Work out the finished part from the listing and answer in its coordinate system (mm). A direction names the side the tool comes from. Coordinates: 2 decimals unless noted, no trailing zeros. Write each loop counter-clockwise with the first axis right and the second up, starting at its lowest first coordinate (ties: lowest second). Pieces come first, ordered by that corner, then holes. Notation, with made-up numbers: (16, 66) - (57, 66) arc R10 ccw to (57, 75) - close; hole circle Ø5 at (62, 3). An arc over 180 degrees is marked (long way). One line per item, written item: value.
Autodesk Inventor part; units mm, degrees
ref_plane "YZ Plane" through (0, 0, 0) normal (1, 0, 0) x (0, 1, 0)
ref_plane "XZ Plane" through (0, 0, 0) normal (0, 1, 0) x (-1, 0, 0)
ref_plane "XY Plane" through (0, 0, 0) normal (0, 0, 1) x (1, 0, 0)
sketch "Sketch1" plane through (0, 0, 0) normal (1, 0, 0) x (0, 1, 0)
  line L0 (22.5733, 37.2966) -> (14.6231, 37.2966)
  line L1 (14.6231, 37.2966) -> (14.6231, 5.5466)
  line L2 (14.6231, 5.5466) -> (22.5733, 5.5466)
  line L3 (22.5733, 5.5466) -> (22.5733, 37.2966)
  point P0 (0, 0)
  dimension "d0" = 7.9502
  dimension "d1" = 31.75
extrude "Extrusion1" add sketch "Sketch1" along normal blind 25.4
sketch "Sketch2" plane through (0, 14.6231, 37.2966) normal (0, 0, 1) x (1, 0, 0)
  line L0 (0, 7.9502) -> (25.4, 7.9502)
  line L1 (25.4, 0) -> (15.24, 0)
  line L2 (15.24, 0) -> (15.24, 7.9502)
  line L3 (15.24, 7.9502) -> (25.4, 7.9502)
  line L4 (25.4, 7.9502) -> (25.4, 0)
  point P0 (0, -14.6231)
  dimension "d4" = 10.16
extrude "Extrusion2" cut sketch "Sketch2" against normal blind 7.62
sketch "Sketch3" plane through (0, 14.6231, 29.6766) normal (0, 0, 1) x (1, 0, 0)
  line L0 (25.4, 7.9502) -> (25.4, 0)
  line L1 (15.24, 7.9502) -> (25.4, 7.9502)
  line L2 (15.24, 0) -> (15.24, 7.9502)
  line L3 (25.4, 0) -> (15.24, 0)
  circle A0 centre (20.32, 3.9502) radius 2
  point P0 (0, -14.6231)
  dimension "d7" = 4
  dimension "d10" = 4
extrude "Extrusion3" cut sketch "Sketch3" against normal blind 2.54 contours A0
sketch "Sketch4" plane through (0, 22.5733, 37.2966) normal (0, 1, 0) x (1, 0, 0)
  circle A0 centre (10.16, 6.0198) radius 2
  line L0 (15.24, 0) -> (15.24, 7.62)
  line L1 (0, 0) -> (15.24, 0)
  point P0 (0, 37.2966)
  dimension "d11" = 4
  dimension "d12" = 5.08
  dimension "d15" = 6.0198
extrude "Extrusion4" cut sketch "Sketch4" against normal blind 25.4
sketch "Sketch5" plane through (0, 22.5733, 37.2966) normal (0, 1, 0) x (1, 0, 0)
  line L0 (0, 0) -> (15.24, 0)
  line L1 (0, 31.75) -> (25.4, 31.75)
  line L2 (14.605, 0) -> (5.715, 0)
  line L3 (5.715, 0) -> (5.715, 31.75)
  line L4 (5.715, 31.75) -> (14.605, 31.75)
  line L5 (14.605, 31.75) -> (14.605, 0)
  circle A0 centre (10.16, 6.0198) radius 2
  point P0 (0, 37.2966)
  point P1 (5.715, 0)
  dimension "d16" = 8.89
  dimension "d17" = 4.445
extrude "Extrusion5" cut sketch "Sketch5" against normal blind 2.54
properties part number "Metal Inside"
Item 1: Determine the mould class of faces 6 (the face through (14.605, 21, 21)), 7 (the face through (3, 22.573, 21)), 8 (the face through (0, 19, 22)) for opening direction X: +X half, -X half, draft (parallel to the pull), parting line (faces both ways), or undercut.
Evaluation:
face 6: undercut
face 7: draft
face 8: -X half
Item 2: Section A-A, the plane x = 10.16 is taken. Determine the outline of the cut face in (y, z).
Evaluation:
outline: (14.62, 5.55) - (20.03, 5.55) - (20.03, 29.28) - (14.62, 29.28) - close; (14.62, 33.28) - (20.03, 33.28) - (20.03, 37.3) - (14.62, 37.3) - close
Item 3: Given pin 1 (3 mm diameter, centred on y = 18, z = 18.5, fed in from -X); pin 2 (5 mm diameter, centred on x = 8.5, z = 10, fed in from +Y); pin 3 (4 mm diameter, centred on x = 20, y = 19.5, fed in from +Z); pin 4 (1.2 mm diameter, centred on x = 19.5, y = 18.5, fed in from +Z), each flat-ended and moving along its own axis, determine where each tip first touches the part or whether it passes through.
Evaluation:
pin 1: stops at x = 0
pin 2: stops at y = 20.03
pin 3: stops at z = 29.68
pin 4: stops at z = 27.14
Item 4: Section C-C, the plane z = 27.5 is taken. Determine the outline of the cut face in (x, y) (3 decimals), then the cut area to 3 significant figures.
Evaluation:
outline: (0, 14.623) - (25.4, 14.623) - (25.4, 22.573) - (14.605, 22.573) - (14.605, 20.033) - (5.715, 20.033) - (5.715, 22.573) - (0, 22.573) - close; hole circle Ø4 at (20.32, 18.573)
area: 167 mm2
Item 5: Section D-D, the plane x = 19.25 is taken. Determine the outline of the cut face in (y, z), then the cut area to 3 significant figures.
Evaluation:
outline: (14.62, 5.55) - (22.57, 5.55) - (22.57, 29.68) - (20.26, 29.68) - (20.26, 27.14) - (16.88, 27.14) - (16.88, 29.68) - (14.62, 29.68) - close
area: 183 mm2
Item 6: Which of the six approach directions +Z, -Z, +X, -X, +Y, -Y give full straight-line access (tool end or side, diameter ignored) to faces 1 (the face through (8, 18, 37.297)), 2 (the face through (19.1, 20.4, 29.677)), 3 (the face through (5.715, 21, 22)), 4 (the face through (20, 19, 27.137)), 5 (the face through (13, 14.623, 22))?
Evaluation:
face 1: +Z, +X, -X, +Y, -Y
face 2: +Z, +X, +Y, -Y
face 3: +Z, -Z, +Y
face 4: +Z
face 5: +Z, -Z, +X, -X, -Y
Item 7: Consider probe 1 along X at (y, z) = (20.25, 9.5) (3 decimals); probe 2 along X at (y, z) = (17, 29.5); probe 3 along Y at (x, z) = (20.32, 28.2). Determine where each line is inside the solid, lowest interval first.
Evaluation:
probe 1: x = 0 to 5.715, 14.605 to 25.4
probe 2: x = 0 to 9.24, 11.08 to 19.09, 21.55 to 25.4
probe 3: y = 14.62 to 16.57, 20.57 to 22.57
Item 8: Section B-B, the plane y = 19 is taken. Determine the outline of the cut face in (x, z).
Evaluation:
outline: (0, 5.55) - (25.4, 5.55) - (25.4, 29.68) - (22.27, 29.68) - (22.27, 27.14) - (18.37, 27.14) - (18.37, 29.68) - (15.24, 29.68) - (15.24, 37.3) - (0, 37.3) - close; hole circle Ø4 at (10.16, 31.28)
